Could you check a few things on this model? Use its own coordinates, in mm. Give positions to 0.01 mm unless a question says otherwise; leave off trailing zeros. Order: outer loops, then holes, each group sorted by start corner. A loop starts at its lowest first (then second) coordinate and runs counter-clockwise, first axis right, second up. Notation, with made-up numbers: (-37, 52) -> (18, 52) arc R29 ccw to (18, 83) -> close; hole circle Ø5 at (-4, 74). An arc over 180 degrees is marked (long way). One line per item, written item: value.
```python
from build123d import *

# Parameters (mm, degrees)
SKETCH_1_W          = 310
SKETCH_1_H          = 310
SKETCH_1_W_2        = 150
SKETCH_1_H_2        = 12
EXTRUDE_1_DEPTH     = 0.8
CUT_EXTRUDE_1_DEPTH = 0.8
FILLET_1_R          = 5


with BuildPart() as part:
    # 草图1 → 凸台-拉伸1 (new body)
    with BuildSketch(Plane.XY):
        with Locations((-24.087837838, -4.538288288)):
            Rectangle(SKETCH_1_W, SKETCH_1_H)
        with Locations((-24.087837838, -165.538288288)):
            Rectangle(SKETCH_1_W_2, SKETCH_1_H_2)
    extrude(amount=EXTRUDE_1_DEPTH)

    # 草图2 → 切除-拉伸1 (cut)
    with BuildSketch(Plane(origin=(0, 0, 0), x_dir=(-1, 0, 0), z_dir=(0, 0, -1))):
        Polygon((99.087837838, -159.538288288), (89.087837838, -171.538288288), (99.087837838, -171.538288288), align=None)
        Polygon((-50.912162162, -159.538288288), (-40.912162162, -171.538288288), (-50.912162162, -171.538288288), align=None)
    extrude(amount=-CUT_EXTRUDE_1_DEPTH, mode=Mode.SUBTRACT)

    # 圆角1
    fillet_1_edges = [part.edges().sort_by_distance(p)[0] for p in [
        (50.912162162, -159.538288288, 0.4),
        (-99.087837838, -159.538288288, 0.4),
        (-89.087837838, -171.538288288, 0.4),
        (40.912162162, -171.538288288, 0.4),
    ]]
    fillet(fillet_1_edges, radius=FILLET_1_R)


solid = part.part
```
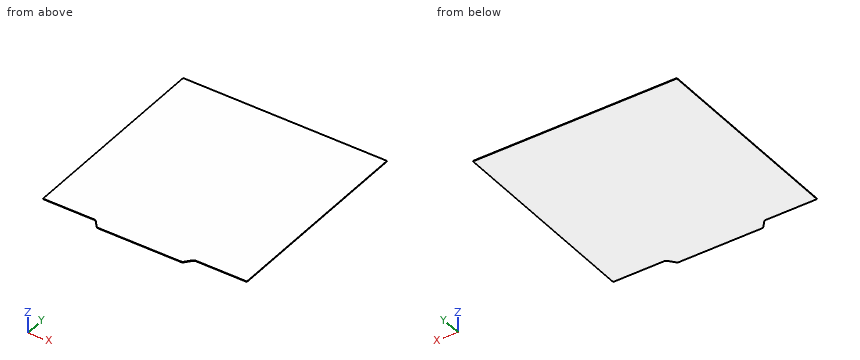
1) Suppose I cut it at B-B, the plane x = 76. Write out the boundary of the cut face in (y, z), then the cut area to 3 significant figures.
Answer below:
outline: (-159.54, 0) -> (150.46, 0) -> (150.46, 0.8) -> (-159.54, 0.8) -> close
area: 248 mm2
2) If I drill on line 1 along Y through (x, z) = (86, 0.7); line 2 along Y through (x, z) = (-89.5, 0.5), over which ranges is the centre line in solid material (lowest first)?
Answer below:
line 1: y = -159.54 to 150.46
line 2: y = -170.71 to 150.46
3) Suppose I cut it at A-A, the plane z = 0.35. Write out the boundary of the cut face in (x, y).
Answer below:
outline: (-179.09, -159.54) -> (-101.43, -159.54) arc R5 cw to (-97.59, -161.34) -> (-90.59, -169.74) arc R5 ccw to (-86.75, -171.54) -> (38.57, -171.54) arc R5 ccw to (42.41, -169.74) -> (49.41, -161.34) arc R5 cw to (53.25, -159.54) -> (130.91, -159.54) -> (130.91, 150.46) -> (-179.09, 150.46) -> close
